Check sheet for the modelled part. Datum: model origin and axes. Units: mm. Coordinates: 2 decimals unless noted, no trailing zeros. Loops run counter-clockwise (first coordinate to the right, second up) from the corner with the lowest first, then second, coordinate; pieces in that order, holes last. Notation, with made-up numbers: (-5, 11.25) - (46, 11.25) arc R19 ccw to (46, 45.25) - close; hole circle Ø8 at (-4, -25.5). An arc over 180 degrees is marked (long way). Answer as a JSON object with one key per item and string values. Group by question number.
from build123d import *

# Parameters (mm, degrees)
BOSS_EXTRUDE1_DEPTH = 10.16
CUT_EXTRUDE1_DEPTH  = 11.16
SKETCH4_W           = 129.547530324
SKETCH4_H           = 444.037072
CUT_EXTRUDE3_DEPTH  = 11.16
SKETCH5_W           = 10.16
SKETCH5_H           = 84.922739191
CUT_EXTRUDE5_DEPTH  = 11.16
CUT_EXTRUDE6_DEPTH  = 11.16
CUT_EXTRUDE7_DEPTH  = 11.16
FILLET1_R           = 19.05


with BuildPart() as part:
    # Sketch1 → Boss-Extrude1 (new body)
    with BuildSketch(Plane.XY):
        with BuildLine():
            Line((20.32, 73.849956434), (0, 73.849956434))
            Line((0, 73.849956434), (0, 10.164894956))
            Line((0, 10.164894956), (20.32, 10.164894956))
            Line((20.32, 10.164894956), (115.06781826, 14.091181531))
            Line((115.06781826, 14.091181531), (115.488322648, 3.943711998))
            Line((115.488322648, 3.943711998), (210.656645296, 7.887423995))
            Line((210.656645296, 7.887423995), (210.236140908, 18.034893528))
            Line((210.236140908, 18.034893528), (305.404463556, 21.978605526))
            Line((305.404463556, 21.978605526), (305.824967945, 11.831135993))
            Line((305.824967945, 11.831135993), (400.993290593, 15.77484799))
            Line((400.993290593, 15.77484799), (400.572786204, 25.922317523))
            Line((400.572786204, 25.922317523), (495.741108852, 29.866029521))
            Line((495.741108852, 29.866029521), (496.161613241, 19.718559988))
            Line((496.161613241, 19.718559988), (591.329935889, 23.662271985))
            Line((591.329935889, 23.662271985), (590.909431501, 33.809741518))
            Line((590.909431501, 33.809741518), (686.077754149, 37.753453516))
            Line((686.077754149, 37.753453516), (686.498258538, 27.605983983))
            Line((686.498258538, 27.605983983), (781.666581186, 31.54969598))
            Line((781.666581186, 31.54969598), (781.246076797, 41.697165514))
            Line((781.246076797, 41.697165514), (781.246076797, 471.95159927))
            ThreePointArc((781.246076797, 471.95159927), (401.049995582, 500.057636465), (20.32, 519.645386783))
            Line((20.32, 519.645386783), (20.32, 455.960325305))
            Line((20.32, 455.960325305), (0, 455.960325305))
            Line((0, 455.960325305), (0, 392.275263826))
            Line((0, 392.275263826), (20.32, 392.275263826))
            Line((20.32, 392.275263826), (20.32, 328.590202348))
            Line((20.32, 328.590202348), (0, 328.590202348))
            Line((0, 328.590202348), (0, 264.905140869))
            Line((0, 264.905140869), (20.32, 264.905140869))
            Line((20.32, 264.905140869), (20.32, 201.220079391))
            Line((20.32, 201.220079391), (0, 201.220079391))
            Line((0, 201.220079391), (0, 137.535017912))
            Line((0, 137.535017912), (20.32, 137.535017912))
            Line((20.32, 137.535017912), (20.32, 73.849956434))
        make_face()
    extrude(amount=BOSS_EXTRUDE1_DEPTH)

    # Sketch2 → Cut-Extrude1 (cut, through all)
    with BuildSketch(Plane.XY.offset(10.16)):
        Polygon((20.32, 471.23904919), (781.246076797, 460.948390721), (781.246076797, 535.017906983), (20.32, 535.017906983), align=None)
    extrude(amount=-CUT_EXTRUDE1_DEPTH, mode=Mode.SUBTRACT)

    # Sketch4 → Cut-Extrude3 (cut, through all)
    with BuildSketch(Plane(origin=(0, 0, 0), x_dir=(-1, 0, 0), z_dir=(0, 0, -1))):
        with Locations((-751.2720237, 249.624519983)):
            Rectangle(SKETCH4_W, SKETCH4_H)
    extrude(amount=-CUT_EXTRUDE3_DEPTH, mode=Mode.SUBTRACT)

    # Sketch5 → Cut-Extrude5 (cut, through all)
    with BuildSketch(Plane(origin=(0, 0, 0), x_dir=(-1, 0, 0), z_dir=(0, 0, -1))):
        Polygon((-686.498258538, 122.676192707), (-686.498258538, 37.753453516), (-686.077754149, 37.753453516), (-676.338258538, 37.753453516), (-676.338258538, 122.676192707), align=None)
        with Locations((-681.418258538, 250.060301493)):
            Rectangle(SKETCH5_W, SKETCH5_H)
        Polygon((-686.498258538, 462.229747042), (-686.498258538, 377.444410279), (-676.338258538, 377.444410279), (-676.338258538, 462.367149469), align=None)
        Polygon((-676.338258538, 37.349855295), (-686.077754149, 37.753453516), (-686.498258538, 27.605983983), (-686.498258538, 26.157835014), (-676.338258538, 26.157835014), align=None)
        Polygon((-686.077754149, 37.753453516), (-686.498258538, 37.753453516), (-686.498258538, 27.605983983), align=None)
        Polygon((-676.338258538, 37.753453516), (-686.077754149, 37.753453516), (-676.338258538, 37.349855295), align=None)
    extrude(amount=-CUT_EXTRUDE5_DEPTH, mode=Mode.SUBTRACT)

    # Sketch9 → Cut-Extrude6 (cut, through all)
    with BuildSketch(Plane(origin=(0, 0, 0), x_dir=(-1, 0, 0), z_dir=(0, 0, -1))):
        Polygon((-20.32, 471.23904919), (-96.513032663, 470.208625209), (-96.375655361, 460.050483081), (-20.32, 461.07904919), align=None)
        Polygon((-172.706065326, 469.178201229), (-172.575642513, 459.019038375), (-248.768675144, 457.988612006), (-248.906065326, 468.147683023), align=None)
    extrude(amount=-CUT_EXTRUDE6_DEPTH, mode=Mode.SUBTRACT)

    # Sketch10 → Cut-Extrude7 (cut, through all)
    with BuildSketch(Plane.XY.offset(10.16)):
        Polygon((323.935601866, 240.017050622), (71.12, 387.534451737), (71.12, 85.442182155), align=None)
        Polygon((589.808964313, 402.575610007), (109.816203442, 409.066965371), (360.851868456, 262.588153871), align=None)
        Polygon((625.538258538, 108.14417143), (625.538258538, 379.763841656), (398.224628495, 240.781222682), align=None)
        Polygon((361.308361904, 218.210119433), (110.294706958, 64.736985613), (590.245383478, 84.62582245), align=None)
    extrude(amount=-CUT_EXTRUDE7_DEPTH, mode=Mode.SUBTRACT)

    # Fillet1
    fillet1_edges = [part.edges().sort_by_distance(p)[0] for p in [
        (398.224628495, 240.781222682, 5.08),
        (625.538258538, 379.763841656, 5.08),
        (625.538258538, 108.14417143, 5.08),
        (109.816203442, 409.066965371, 5.08),
        (589.808964313, 402.575610007, 5.08),
        (360.851868456, 262.588153871, 5.08),
        (361.308361904, 218.210119433, 5.08),
        (590.245383478, 84.62582245, 5.08),
        (110.294706958, 64.736985613, 5.08),
        (71.12, 387.534451737, 5.08),
        (323.935601866, 240.017050622, 5.08),
        (71.12, 85.442182155, 5.08),
    ]]
    fillet(fillet1_edges, radius=FILLET1_R)


solid = part.part
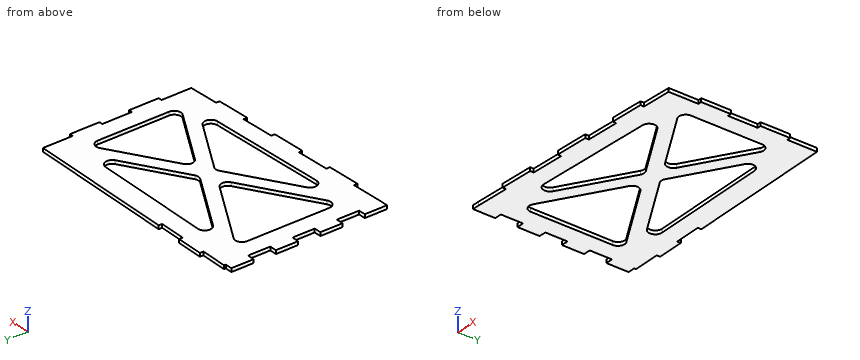
1. Sectioned sample at A-A on y = 175.5. Record the cut outline in (x, z), plus the area to 3 significant figures.
2. Sectioned sample at B-B on x = 80. Record the cut outline in (y, z), plus the area to 3 significant figures.
3. Material ranges on line 1 (X direction, y = 240.5, z = 4.5); line 2 (X direction, y = 153, z = 6.75); line 3 (X direction, y = 325, z = 8.25), recorded low to high.
4. Sectioned sample at C-C on x = 516.5. Record the cut outline in (y, z).
5. Sectioned sample at D-D on z = 8. State how many separate pieces and enclosed holes the cut face has, plus the area to 3 significant figures.
6. Gauge pin test, flat ends, axial feed: pin 1 (5 mm diameter, centred on x = 680, z = 3, fed in from -Y); pin 2 (6 mm diameter, centred on x = 177.5, z = 2, fed in from -Y); pin 3 (1.5 mm diameter, centred on x = 437, z = 9, fed in from +Y). Record the tip position at first contact, or that the pin passes through.
Answers follow:
{
 "1": {"outline": "(0, 0) - (71.12, 0) - (71.12, 10.16) - (0, 10.16) - close; (218.41, 0) - (291.45, 0) - (291.45, 10.16) - (218.41, 10.16) - close; (434.51, 0) - (510.1, 0) - (510.1, 10.16) - (434.51, 10.16) - close; (625.54, 0) - (686.5, 0) - (686.5, 10.16) - (625.54, 10.16) - close", "area": "2,850 mm^2"},
 "2": {"outline": "(12.64, 0) - (103.31, 0) - (103.31, 10.16) - (12.64, 10.16) - close; (370.47, 0) - (460.27, 0) - (460.27, 10.16) - (370.47, 10.16) - close", "area": "1,830 mm^2"},
 "3": {"line 1": "x = 20.32 to 71.12, 305.82 to 416.33, 625.54 to 676.34", "line 2": "x = 0 to 71.12, 181.61 to 254.65, 473.07 to 548.66, 625.54 to 686.5", "line 3": "x = 0 to 71.12, 178.29 to 253.89, 462.93 to 535.97, 625.54 to 686.5"},
 "4": {"outline": "(20.56, 0) - (81.57, 0) - (81.57, 10.16) - (20.56, 10.16) - close; (127.66, 0) - (171.77, 0) - (171.77, 10.16) - (127.66, 10.16) - close; (313.1, 0) - (357.75, 0) - (357.75, 10.16) - (313.1, 10.16) - close; (403.57, 0) - (464.53, 0) - (464.53, 10.16) - (403.57, 10.16) - close"},
 "5": {"separate pieces": "1", "enclosed holes": "4", "area": "166,000 mm^2"},
 "6": {"pin 1": "stops at y = 122.68", "pin 2": "stops at y = 6.39", "pin 3": "stops at y = 465.61"}
}
